Input: part model. Units: mm. Frame: model coordinates. A direction names the side the tool comes from. Give positions to 0.01 mm unless a question says otherwise; leave off trailing zeros. Write each loop counter-clockwise with the first axis right and the second up, starting at its lowest first coordinate (ties: lowest second). Pieces come first, ordered by that corner, then holes. Notation, with made-up numbers: (21.25, -6.5) - (56.25, -6.5) arc R19 cw to (56.25, 25.5) - close; hole circle Ø5 at (67.25, 82.5). An arc over 180 degrees is marked (long way). Answer as CSV lines item,"result".
Autodesk Inventor part; units mm, degrees
ref_plane "YZ Plane" through (0, 0, 0) normal (1, 0, 0) x (0, 1, 0)
ref_plane "XZ Plane" through (0, 0, 0) normal (0, 1, 0) x (-1, 0, 0)
ref_plane "XY Plane" through (0, 0, 0) normal (0, 0, 1) x (1, 0, 0)
sketch "Sketch1" plane through (0, 0, 0) normal (0, 0, 1) x (1, 0, 0)
  line L0 (0, 0) -> (0, -3)
  line L1 (0, -3) -> (7, -3)
  line L2 (7, -3) -> (7, 0)
  line L3 (0, 0) -> (-22, 0)
  line L4 (-22, 0) -> (-22, -3)
  line L5 (-22, -3) -> (0, -3)
  line L6 (0, -3) -> (0, 0)
  line L7 (-22, 0) -> (-32, 0)
  line L8 (-32, 0) -> (-32, -3)
  line L9 (-32, -3) -> (-22, -3)
  line L10 (-22, -3) -> (-22, 0)
  line L11 (-32, 0) -> (7, 0)
  line L12 (7, 0) -> (7, -70)
  line L13 (7, -70) -> (-32, -70)
  line L14 (-32, -70) -> (-32, 0)
  circle A0 centre (7, -70) radius 10
  point P0 (-3, -70)
  point P1 (7, -60)
  dimension "d0" = 3
  dimension "d1" = 7
  dimension "d2" = 22
  dimension "d3" = 3
  dimension "d4" = 10
  dimension "d5" = 3
  dimension "d6" = 39
  dimension "d7" = 70
  dimension "d8" = 20
extrude "Extrusion1" add sketch "Sketch1" along normal blind 3 contours L0 L5 L4 L3 | L1 L12 A0 L13 L14 L9 L5
mirror "Mirror1" about plane through (-32, -70, 0) normal (0, -1, 0) of "Extrusion1"
sketch "Sketch2" plane through (-32, -3, 0) normal (-1, 0, 0) x (0, 0, 1)
  line L0 (0, 0) -> (3, 0)
  line L1 (3, 0) -> (3, -17)
  line L2 (3, -17) -> (0, -17)
  line L3 (0, -17) -> (0, 0)
  line L4 (3, -17) -> (0, -17)
  line L5 (0, -17) -> (0, -37)
  line L6 (0, -37) -> (3, -37)
  line L7 (3, -37) -> (3, -17)
  line L8 (0, -37) -> (3, -37)
  line L9 (3, -37) -> (3, -57)
  line L10 (3, -57) -> (0, -57)
  line L11 (0, -57) -> (0, -37)
  point P0 (0, 3)
  dimension "d11" = 3
  dimension "d12" = 17
  dimension "d13" = 3
  dimension "d14" = 20
  dimension "d15" = 3
  dimension "d16" = 20
extrude "Extrusion2" add sketch "Sketch2" along normal blind 3 contours L2 L7 L6 L5
sketch "Sketch3" plane through (-32, -137, 0) normal (-1, 0, 0) x (0, 0, 1)
  line L0 (0, 97) -> (3, 97)
  line L1 (3, 97) -> (3, 77)
  line L2 (3, 77) -> (0, 77)
  line L3 (0, 77) -> (0, 97)
  line L4 (3, 77) -> (0, 77)
  line L5 (0, 77) -> (0, 57)
  line L6 (0, 57) -> (3, 57)
  line L7 (3, 57) -> (3, 77)
  line L8 (0, 97) -> (0, 0)
  line L9 (3, 57) -> (0, 57)
  line L10 (0, 57) -> (0, 37)
  line L11 (0, 37) -> (3, 37)
  line L12 (3, 37) -> (3, 57)
  point P0 (0, 137)
  dimension "d19" = 3
  dimension "d20" = 20
  dimension "d21" = 3
  dimension "d22" = 20
  dimension "d23" = 20
extrude "Extrusion3" add sketch "Sketch3" along normal blind 3 contours L2 L7 L6 L5
sketch "Sketch4" plane through (-32, -137, 0) normal (-1, 0, 0) x (0, 0, 1)
  line L0 (2.7004, 57) -> (3, 37.0022)
  line L1 (3, 57) -> (3, 0)
  line L2 (0, 57) -> (0, 0)
  line L3 (3, 37.0022) -> (0, 37.0022)
  line L4 (0, 37.0022) -> (0, 17.0022)
  line L5 (0, 17.0022) -> (3, 17.0022)
  line L6 (3, 17.0022) -> (3, 37.0022)
  point P0 (0, 137)
  point P1 (3, 17.0022)
  point P2 (0, 37.0022)
  dimension "d26" = 20
  dimension "d27" = 20
extrude "Extrusion4" add sketch "Sketch4" along normal blind 3
properties part number "ACHTERKANT"
Item 1: Ray query, line 1 (X direction, y = -98.5, z = 1.15); line 2 (Y direction, x = -2, z = 1.85); line 3 (Y direction, x = -28, z = 0.7). Return the intervals inside material, ascending. Write a range as from..to.
The answers:
line 1,"-32..7"
line 2,"-140..-74.36, -65.64..0"
line 3,"-137..-3"
Item 2: Cut plane B-B on z = 1. Return the cut outline in (x, y), plus the area to 3 significant figures.
The answers:
outline,"(-35, -120) - (-32, -120) - (-32, -137) - (-22, -137) - (-22, -140) - (0, -140) - (0, -137) - (7, -137) - (7, -80) arc R10 cw to (7, -60) - (7, -3) - (0, -3) - (0, 0) - (-22, 0) - (-22, -3) - (-32, -3) - (-32, -20) - (-35, -20) - (-35, -40) - (-32, -40) - (-32, -60) - (-35, -60) - (-35, -80) - (-32, -80) - (-32, -100) - (-35, -100) - close"
area,"5,380 mm²"
Item 3: Reachability of faces 1 (the face through (-33, -99.998, 2)), 2 (the face through (0, -138, 1)), 3 (the face through (-27, -137, 1)), 4 (the face through (0, -1, 1)), 5 (the face through (-32, -12, 1)) from +Z, -Z, +X, -X, +Y, -Y: full face, straight path, thin tool, end or side. Return the list, or none.
The answers:
face 1,"+Z, -Z, -X"
face 2,"+Z, -Z, +X, -Y"
face 3,"+Z, -Z, -X, -Y"
face 4,"+Z, -Z, +X, +Y"
face 5,"+Z, -Z, -X, +Y"
Item 4: Contact query for flat-ended pins moving along their axis: pin 1 (1.5 mm diameter, centred on y = -128, z = 1.5, fed in from -X); pin 2 (0.9 mm diameter, centred on x = -34, z = 2, fed in from -Y); pin 3 (1.5 mm diameter, centred on x = -33.5, z = 1, fed in from +Y). Output: stop coordinate, or through.
The answers:
pin 1,"x = -32"
pin 2,"y = -120"
pin 3,"y = -20"
Item 5: Cut plane C-C on y = -70. Return the cut outline in (x, z).
The answers:
outline,"(-35, 0) - (-3, 0) - (-3, 3) - (-35, 3) - close"
Item 6: Mould query, pull axis Y, two halves, no side actions, for faces 6 (the face through (-33, -119.998, 1)), 7 (the face through (-27, -3, 1)), 8 (the face through (-32, -50, 1)). Classes: +Y half, -Y half, draft (parallel to the pull), parting line (faces both ways), or undercut.
The answers:
face 6,"-Y half"
face 7,"+Y half"
face 8,"undercut"
Item 7: Cut plane A-A on x = -1.5. Return the cut outline in (y, z).
The answers:
outline,"(-140, 0) - (-75.27, 0) - (-75.27, 3) - (-140, 3) - close; (-64.73, 0) - (0, 0) - (0, 3) - (-64.73, 3) - close"
